CAD build for the part. Positions are in the model's coordinates, mm. Round coordinates to 2 decimals unless told otherwise and drop trailing zeros. Order: outer loops, then holes, each group sorted by start corner. A loop starts at its lowest first (then second) coordinate and runs counter-clockwise, first axis right, second up. Notation, with made-up numbers: (32.25, 58) -> (83.25, 58) arc R13 ccw to (83.25, 83) -> close; hole circle Ø1 at (-38, 13.25). An arc over 180 degrees is marked (long way). Return JSON: item names as keys, results as strings. Group by question number.
Q1. Cut at B-B (y = 313). Write the cut outline in (x, z) (3 decimals), then the cut area to 3 significant figures.
Q2. Cut at A-A (y = 89). Write the cut outline in (x, z).
Q3. Probe line 1 along Z through (x, y) = (546, 375.5); line 2 along Z through (x, y) = (548.5, 404); line 3 along X through (y, z) = (509.5, -434). List the from-to ranges inside material, lowest first.
Q4. Flat gauge pins, fed straight in: pin 1 (12 mm diameter, centred on x = 486, y = 666, fed in from -Z); pin 2 (8.5 mm diameter, centred on x = -24, z = -695, fed in from -Y); pin 3 (6 mm diameter, centred on y = 429.5, z = -611, fed in from -X). Where does each tip first touch, or does it go through?
Q5. Cut at D-D (x = 238.5). Write the cut outline in (y, z).
Q6. Cut at C-C (y = 603). Write the cut outline in (x, z) (3 decimals), then the cut area to 3 significant figures.
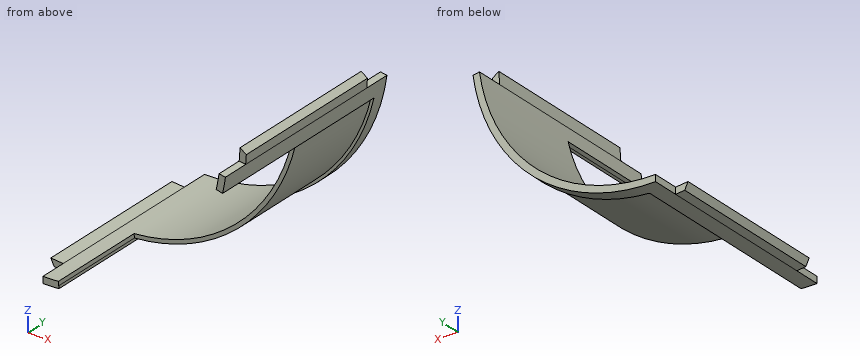
from build123d import *

# Parameters (mm, degrees)
EXTRUDE_1_DEPTH       = 800
EXTRUDE_2_DEPTH       = 300
MIRROR_3_COPY_1_DEPTH = 300
MIRROR_3_COPY_2_DEPTH = 300
CUT_EXTRUDE_1_DEPTH   = 750
CUT_EXTRUDE_2_DEPTH   = 375


with BuildPart() as part:
    # 草图1 → 凸台-拉伸1 (new body)
    with BuildSketch(Plane(origin=(0, 0, 0), x_dir=(1, 0, 0), z_dir=(0, 1, 0))):
        with BuildLine():
            Line((0, 705), (0, 680))
            ThreePointArc((0, 680), (446.120139714, 513.202514551), (673.382286744, 94.637708653))
            Line((673.382286744, 94.637708653), (698.138988463, 98.117036177))
            ThreePointArc((698.138988463, 98.117036177), (462.521615438, 532.070254057), (0, 705))
        make_face()
    extrude(amount=EXTRUDE_1_DEPTH)

    # 草图2 → 凸台-拉伸2 (add)
    with BuildSketch(Plane(origin=(0, 400, 0), x_dir=(1, 0, 0), z_dir=(0, 1, 0))):
        Polygon((698.138988463, 98.117036177), (673.382286744, 94.637708653), (676.691143372, 47.318854326), (700.56509889, 63.422040654), align=None)
    extrude_2 = extrude(amount=-EXTRUDE_2_DEPTH)

    # 镜向1: 凸台-拉伸2 across plane
    add(extrude_2.mirror(Plane(origin=(446.120139714, 800, -513.202514551), x_dir=(-0.6560590289905062, 0, 0.754709580222773), z_dir=(-0.7547095802227732, 0, -0.656059028990506))))

    # 镜向2: 凸台-拉伸2 across plane
    add(extrude_2.mirror(Plane.ZX.offset(400)))

    # 镜向3 copy 1 sketch → 镜向3 copy 1 (add)
    with BuildSketch(Plane(origin=(0, 400, 0), x_dir=(-0.13917310096006918, 0, -0.99026806874157), z_dir=(0, -1, 0))):
        Polygon((698.138988463, 98.117036177), (673.382286744, 94.637708653), (676.691143372, 47.318854326), (700.56509889, 63.422040654), align=None)
    extrude(amount=-MIRROR_3_COPY_1_DEPTH)

    # 镜向3 copy 2 sketch → 镜向3 copy 2 (add)
    with BuildSketch(Plane(origin=(0, 400, 0), x_dir=(-0.13917310096006918, 0, -0.99026806874157), z_dir=(0, 1, 0))):
        Polygon((698.138988463, -98.117036177), (673.382286744, -94.637708653), (676.691143372, -47.318854326), (700.56509889, -63.422040654), align=None)
    extrude(amount=-MIRROR_3_COPY_2_DEPTH)

    # 草图4 → 切除-拉伸1 (cut)
    with BuildSketch(Plane.XZ):
        with BuildLine():
            Line((677.274077507, -155.96417517), (687.019028263, -158.208264022))
            ThreePointArc((687.019028263, -158.208264022), (462.521615438, -532.070254057), (61.05402349, -702.351341008))
            Line((61.05402349, -702.351341008), (60.188008972, -692.388910639))
            ThreePointArc((60.188008972, -692.388910639), (455.961025148, -524.523158255), (677.274077507, -155.96417517))
        make_face()
    extrude(amount=-CUT_EXTRUDE_1_DEPTH, mode=Mode.SUBTRACT)

    # 草图5 → 切除-拉伸2 (cut)
    with BuildSketch(Plane.XZ):
        with BuildLine():
            Line((677.274077507, -155.96417517), (662.656651374, -152.598041893))
            ThreePointArc((662.656651374, -152.598041893), (446.120139714, -513.202514551), (58.888987196, -677.445265086))
            Line((58.888987196, -677.445265086), (60.188008972, -692.388910639))
            ThreePointArc((60.188008972, -692.388910639), (455.961025148, -524.523158255), (677.274077507, -155.96417517))
        make_face()
    extrude(amount=-CUT_EXTRUDE_2_DEPTH, mode=Mode.SUBTRACT)


solid = part.part
Solution:
{
 "1": {"outline": "(-47.319, -676.691) -> (-34.695, -702.574) -> (0, -705) arc R705 ccw to (61.054, -702.351) -> (58.889, -677.445) arc R680 cw to (0, -680) -> close; (662.657, -152.598) -> (687.019, -158.208) arc R705 ccw to (698.139, -98.117) -> (700.565, -63.422) -> (676.691, -47.319) -> (673.382, -94.638) arc R680 cw to start", "area": "5,050 mm²"},
 "2": {"outline": "(0, -705) arc R705 ccw to (61.05, -702.35) -> (58.89, -677.45) arc R680 cw to (0, -680) -> close; (662.66, -152.6) -> (687.02, -158.21) arc R705 ccw to (698.14, -98.12) -> (673.38, -94.64) arc R680 cw to start"},
 "3": {"line 1": "z = -430.01 to -405.32", "line 2": "z = -426.82 to -401.93", "line 3": "x = 523.49 to 542.83"},
 "4": {"pin 1": "stops at z = -502.62", "pin 2": "stops at y = 100", "pin 3": "stops at x = 292.24"},
 "5": {"outline": "(375, -652.8) -> (750, -652.8) -> (750, -663.43) -> (800, -663.43) -> (800, -636.8) -> (375, -636.8) -> close"},
 "6": {"outline": "(-47.319, -676.691) -> (-34.695, -702.574) -> (0, -705) arc R705 ccw to (61.054, -702.351) -> (60.188, -692.389) arc R695 ccw to (677.274, -155.964) -> (687.019, -158.208) arc R705 ccw to (698.139, -98.117) -> (700.565, -63.422) -> (676.691, -47.319) -> (673.382, -94.638) arc R680 cw to (0, -680) -> close", "area": "18,000 mm²"}
}
